from build123d import *

# Parameters (mm, degrees)
F0_W     = 152.4
F0_H     = 76.2
F1_DEPTH = 6.35
F2_W     = 3.175
F2_H     = 2.54
F3_DEPTH = 152.4
F4_W     = 3.175
F4_H     = 2.54
F5_DEPTH = 152.4


with BuildPart() as f1:
    # F0 (on Right) → F1 (new body)
    with BuildSketch(Plane.YZ):
        Rectangle(F0_W, F0_H)
    extrude(amount=F1_DEPTH)

    # F2 (on face) → F3 (cut)
    with BuildSketch(Plane(origin=(0, 0, -38.1), x_dir=(1, 0, 0), z_dir=(0, 0, -1))):
        with Locations((4.7625, 74.93)):
            Rectangle(F2_W, F2_H)
    extrude(amount=-F3_DEPTH, mode=Mode.SUBTRACT)

    # F4 (on face) → F5 (cut)
    with BuildSketch(Plane(origin=(0, 0, -38.1), x_dir=(1, 0, 0), z_dir=(0, 0, -1))):
        with Locations((4.7625, -74.93)):
            Rectangle(F4_W, F4_H)
    extrude(amount=-F5_DEPTH, mode=Mode.SUBTRACT)


solid = f1.part
Here's how the part is built. I have some questions about the finished solid (model axes, mm). A direction names the side the tool comes from. Round coordinates to 2 decimals unless told otherwise and drop trailing zeros. Order: outer loops, then holes, each group sorted by start corner. A loop starts at its lowest first (then second) coordinate and runs counter-clockwise, first axis right, second up. Notation, with made-up numbers: (11.5, -26) -> (16.5, -26) arc R23 ccw to (16.5, -3) -> close; hole circle Ø1 at (59.25, -1). An arc over 180 degrees is marked (long way). Return JSON: item names as keys, results as strings.
Q1. I need wall thicknesses on line 1 along Y through (x, z) = (5.5, -21). Which ranges of the line are inside material? Lowest first, please. Write a range as from..to.
Filled sheet:
{"line 1": "y = -73.66..73.66"}
Q2. Which directions (+Z, -Z, +X, -X, +Y, -Y) give clear straight access to the entire face, cutting with the end or side of a thin tool? Please do faces 1 (the flat face through (3, -1, 38.1)), 2 (the flat face through (5, -73.66, -1)), 3 (the flat face through (5, 73.66, -1)).
Filled sheet:
{"face 1": "+Z, +X, -X, +Y, -Y", "face 2": "+Z, -Z, +X, -Y", "face 3": "+Z, -Z, +X, +Y"}
Q3. If we section it at A-A on z = -20.5: List the corners of the cut face in (x, y) for me (3 decimals).
Filled sheet:
{"outline": "(0, -76.2) -> (3.175, -76.2) -> (3.175, -73.66) -> (6.35, -73.66) -> (6.35, 73.66) -> (3.175, 73.66) -> (3.175, 76.2) -> (0, 76.2) -> close"}
Q4. For pin 1 Ø0.8 at (y, z) = (-74.5, -13.5) entering from +X (3 decimals); pin 2 Ø1 at (x, z) = (4.5, -1.5) entering from +Y, each with a flat end and sliding along its axis, tell me the tip position at first contact or that it passes through.
Filled sheet:
{"pin 1": "stops at x = 3.175", "pin 2": "stops at y = 73.66"}
